Input: part model. Units: mm. Frame: model coordinates. A direction names the side the tool comes from. Round coordinates to 2 decimals unless told otherwise and drop trailing zeros. Order: outer loops, then holes, each group sorted by start corner. A loop starts at its lowest first (then second) coordinate and runs counter-clockwise, first axis right, second up. Notation, with made-up numbers: (7, 35) - (39, 35) arc R20 cw to (39, 62) - close; hole circle Ø3 at (25, 0.25). An arc over 180 degrees is marked (long way). One line per item, written item: value. Start each with the question number.
from build123d import *

# Parameters (mm, degrees)
CYLINDER019_R             = 17
CYLINDER019_DEPTH         = 14
CYLINDER020_R             = 5.5
CYLINDER020_DEPTH         = 6
CYLINDER018_R             = 17
CYLINDER018_DEPTH         = 30
BOX003_W                  = 11
BOX003_H                  = 10
BOX003_DEPTH              = 21
CYLINDER021_R             = 3
CYLINDER021_DEPTH         = 15
CYLINDER017_R             = 18.4
CYLINDER017_DEPTH         = 20
FUSION003_ROLL_ANGLE      = 90
FUSION003_PLACEMENT_ANGLE = 180


with BuildPart() as encoder002:
    # Cylinder019 → Cylinder019 (new body)
    with BuildSketch(Plane(origin=(0, -298, 0), x_dir=(1, 0, 0), z_dir=(0, 0, 1))):
        Circle(CYLINDER019_R)
    extrude(amount=CYLINDER019_DEPTH)


with BuildPart() as cilindro004:
    # Cylinder020 → Cylinder020 (new body)
    with BuildSketch(Plane(origin=(0, -292, 64), x_dir=(1, 0, 0), z_dir=(0, 0, 1))):
        Circle(CYLINDER020_R)
    extrude(amount=CYLINDER020_DEPTH)


with BuildPart() as motor002:
    # Cylinder018 → Cylinder018 (new body)
    with BuildSketch(Plane(origin=(0, -298, 14), x_dir=(1, 0, 0), z_dir=(0, 0, 1))):
        Circle(CYLINDER018_R)
    extrude(amount=CYLINDER018_DEPTH)


with BuildPart() as cubo002:
    # Box003 → Box003 (new body)
    with BuildSketch(Plane(origin=(2, -191, -2), x_dir=(1, 0, 0), z_dir=(0, 0, 1))):
        with Locations((5.5, 5)):
            Rectangle(BOX003_W, BOX003_H)
    extrude(amount=BOX003_DEPTH)


with BuildPart() as cut002:
    # Cylinder021 → Cylinder021 (new body)
    with BuildSketch(Plane(origin=(0, -186, 0), x_dir=(1, 0, 0), z_dir=(0, 0, 1))):
        Circle(CYLINDER021_R)
    extrude(amount=CYLINDER021_DEPTH)

    # Cut002: cut Cubo002
    add(cubo002.part, mode=Mode.SUBTRACT)


with BuildPart() as cut002_1:
    # Cut002 placement: moved
    add(cut002.part.moved(Location((0, -106, 70))))


with BuildPart() as obj1:
    # Cylinder017 → Cylinder017 (new body)
    with BuildSketch(Plane(origin=(0, -298, 44), x_dir=(1, 0, 0), z_dir=(0, 0, 1))):
        Circle(CYLINDER017_R)
    extrude(amount=CYLINDER017_DEPTH)

    # Fusion003: union Encoder002, Cilindro004, Motor002, Cut002
    add(encoder002.part)
    add(cilindro004.part)
    add(motor002.part)
    add(cut002_1.part)


with BuildPart() as obj1_1:
    # Fusion003 roll: moved
    add(obj1.part.rotate(Axis((0, 0, 0), (1, 0, 0)), FUSION003_ROLL_ANGLE))


with BuildPart() as obj1_2:
    # Fusion003 placement: moved
    add(obj1_1.part.moved(Location((43, 75, 283))).rotate(Axis((43, 75, 283), (0, 0, 1)), FUSION003_PLACEMENT_ANGLE))


solid = obj1_2.part
Item 1: Section query C-C on y = 142.5. Return loops of the section in (x, z).
Item 2: Section query A-A on x = 43. Return loops of the section in (y, z).
Item 3: Line query: L1, parallel to Z at x = 43.5, y = 83.5; L2, parallel to Y at x = 44, z = -31; L3, parallel to Z at x = 46.5, y = 95. Output: solid intervals per line, ascending.
Item 4: Section query D-D on z = 1. Return loops of the section in (x, y), and give its area (3 significant figures).
Item 5: Reachability of faces 1 (the face through (37.6, 119, -31.3)), 2 (the face through (41, 152, -9)), 3 (the face through (46, 152, -9)), 4 (the face through (43, 75, -15)) from +Z, -Z, +X, -X, +Y, -Y: full face, straight path, thin tool, end or side. Return the list, or none.
Item 6: First-contact query: pin 1 Ø3.5 at (y, z) = (155.5, -9) entering from -X; pin 2 Ø1 at (x, y) = (34.5, 98.5) entering from +Z; pin 3 Ø4 at (y, z) = (119, -28) entering from -X. Flat tips, straight axial feed; report the tip coordinate or a pass-through.
Item 7: Section query B-B on z = -18.5. Return loops of the section in (x, y).
Geometry results:
1. outline: circle Ø11 at (43, -9)
2. outline: (75, -32) - (119, -32) - (119, -33.4) - (139, -33.4) - (139, -14.5) - (145, -14.5) - (145, -12) - (160, -12) - (160, -6) - (145, -6) - (145, -3.5) - (139, -3.5) - (139, 3.4) - (119, 3.4) - (119, 2) - (75, 2) - close
3. L1: z = -31.99 to 1.99
3. L2: y = 75 to 139
3. L3: z = -31.64 to 1.64
4. outline: (33.91, 119) - (37.26, 119) - (37.26, 75) - (48.74, 75) - (48.74, 119) - (52.09, 119) - (52.09, 139) - (33.91, 139) - close
4. area: 869 mm^2
5. face 1: -Y
5. face 2: +Z, -Z, -X, +Y
5. face 3: +Y
5. face 4: +Z, -Z, +X, -X, -Y
6. pin 1: stops at x = 41
6. pin 2: stops at z = 0
6. pin 3: stops at x = 28.25
7. outline: (24.94, 119) - (26.36, 119) - (26.36, 75) - (59.64, 75) - (59.64, 119) - (61.06, 119) - (61.06, 139) - (24.94, 139) - close
